Model file for the job. Use its own axes, mm. A direction names the side the tool comes from. Coordinates: 2 decimals unless noted, no trailing zeros. Write each loop counter-clockwise with the first axis right and the second up, starting at its lowest first coordinate (ties: lowest second). Pieces come first, ordered by that corner, then holes. Notation, with made-up numbers: (-7, 73.25) -> (-1, 73.25) arc R25 cw to (-1, 107.25) -> close; hole circle Ø9 at (59.5, 37.25). An arc over 180 degrees is marked (long way). Answer as a JSON object with one key per item and string values. Group by question number.
from build123d import *

# Parameters (mm, degrees)
SKETCH1_R           = 12.7
BOSS_EXTRUDE1_DEPTH = 50.8
SKETCH2_R           = 11.43
BOSS_EXTRUDE2_DEPTH = 19.05
SKETCH4_R           = 9.525
BOSS_EXTRUDE3_DEPTH = 12.7
FILLET1_R           = 5.08
CUT_EXTRUDE1_DEPTH  = 9.525


with BuildPart() as part:
    # Sketch1 → Boss-Extrude1 (new body)
    with BuildSketch(Plane.XY):
        Circle(SKETCH1_R)
    extrude(amount=BOSS_EXTRUDE1_DEPTH)

    # Sketch2 → Boss-Extrude2 (add)
    with BuildSketch(Plane.XY.offset(50.8)):
        with Locations(Location((0, 0, 0), (0, 0, 180))):
            Circle(SKETCH2_R)
    extrude(amount=BOSS_EXTRUDE2_DEPTH)

    # Sketch4 → Boss-Extrude3 (add)
    with BuildSketch(Plane.XY.offset(69.85)):
        Circle(SKETCH4_R)
    extrude(amount=BOSS_EXTRUDE3_DEPTH)

    # Fillet1
    # the kernel refuses this fillet: 5.08 mm, written as the material it adds along each edge
    with BuildSketch(Plane(origin=(0, 0, 69.85), x_dir=(1, 0, 0), z_dir=(0, -1, 0))) as fillet1_piece_1:
        with BuildLine():
            CenterArc((14.605, 3.965573729), FILLET1_R, 180, 51.317812547)
            Line((9.525, 3.965573729), (9.4234, 3.965573729))
            Line((9.4234, 3.965573729), (9.4234, 0))
            Line((9.4234, 0), (9.525, -0.1016))
            ThreePointArc((9.525, -0.1016), (10.4775, -0.1016), (11.3665, -0.079311475))
            Line((11.3665, -0.079311475), (11.43, 0))
        make_face()
    revolve(axis=Axis((0, 0, 69.85), (0, 0, 1)))

    # Sketch5 → Cut-Extrude1 (cut)
    with BuildSketch(Plane.XY.offset(82.55)):
        Polygon((3.698041146, 6.33149469), (-3.634214672, 6.368344922), (-7.332255819, 0.036850232), (-3.698041146, -6.33149469), (3.634214672, -6.368344922), (7.332255819, -0.036850232), align=None)
    extrude(amount=-CUT_EXTRUDE1_DEPTH, mode=Mode.SUBTRACT)


solid = part.part
(1) Cut at B-B on z = 22.5. List the corners of the cut face in (x, y), plus the area to 3 significant figures.
(2) Cut at A-A on x = 0. List the corners of the cut face in (y, z) (3 decimals).
(3) Pull direction X, two halves, no side cores. Call faces 1 (the face through (5.457, -3.247, 77.854)), 2 (the face through (9.07, 6.955, 60.192)), 3 (the face through (0, 0, 0)): released by +X, released by -X, zero draft, split by the parting line, or undercut.
(4) Cut at C-C on z = 66. List the corners of the cut face in (x, y).
(5) Pin check, flat tips, straight feed: pin 1 (3 mm diameter, centred on y = -10, z = 27, fed in from -X); pin 2 (12 mm diameter, centred on x = 5.5, z = 71, fed in from -Y); pin 3 (2 mm diameter, centred on x = -2.5, z = 32.5, fed in from -Y). Stop position of each tip, or through.
(6) Wall check: probe 1 along Y at (x, z) = (0.5, 29); probe 2 along Z at (x, y) = (-6.25, -11). Give the ranges that are in metal, low to high.
(7) 3-axis set-ups, long thin cutter, end or side, ignore diameter. For faces 4 (the face through (-2.75, -12.4, 25.04)), 5 (the face through (0, 0, 73.025)): which of +Z, -Z, +X, -X, +Y, -Y reach the whole face in a straight line?
Results found:
{
 "1": {"outline": "circle Ø25.4 at (0, 0)", "area": "507 mm²"},
 "2": {"outline": "(-12.7, 0) -> (12.7, 0) -> (12.7, 50.8) -> (11.43, 50.8) -> (11.43, 69.85) arc R5.08 cw to (9.525, 73.816) -> (9.525, 82.55) -> (6.35, 82.55) -> (6.35, 73.025) -> (-6.35, 73.025) -> (-6.35, 82.55) -> (-9.525, 82.55) -> (-9.525, 73.816) arc R5.08 cw to (-11.43, 69.85) -> (-11.43, 50.8) -> (-12.7, 50.8) -> close"},
 "3": {"face 1": "undercut", "face 2": "split by the parting line", "face 3": "zero draft"},
 "4": {"outline": "circle Ø22.86 at (0, 0)"},
 "5": {"pin 1": "stops at x = -9.44", "pin 2": "stops at y = -11.43", "pin 3": "stops at y = -12.61"},
 "6": {"probe 1": "y = -12.69 to 12.69", "probe 2": "z = 0 to 50.8"},
 "7": {"face 4": "+Z, -Z", "face 5": "+Z"}
}
